Geometry check sheet. Reference: the model listing, model coordinates, mm. A direction names the side the tool comes from. Give positions to 0.01 mm unless a question says otherwise; leave off trailing zeros. Loops run counter-clockwise (first coordinate to the right, second up) from the corner with the lowest first, then second, coordinate; pieces in that order, holes last.
1. Material ranges on L1, parallel to X at y = -34.5, z = 36.65; L2, parallel to X at y = -30.5, z = 7; L3, parallel to Z at x = 5, y = -35, recorded low to high.
2. Cross-section at D-D, the plane y = -4. Record the cut outline in (x, z), plus the area to 3 significant figures.
3. Go/stop test with flat-tipped pins: pin 1 Ø1 at (y, z) = (-33.5, 37) entering from -X; pin 2 Ø2.5 at (x, z) = (36.65, 36.65) entering from +Y. Record where each tip stops, or that it passes through.
4. Cross-section at B-B, the plane z = 21.15. Record the cut outline in (x, y), plus the area to 3 significant figures.
5. Cross-section at C-C, the plane x = 33.5. Record the cut outline in (y, z).
6. Cross-section at A-A, the plane y = -35.5. Record the cut outline in (x, z).
7. Tool access check on faces 4 (the flat face through (0, -19, 21)), 5 (the cylindrical face through (13.04, -39.49, 28.58)). Record the directions out of +Z, -Z, +X, -X, +Y, -Y that give a thin tool (end or side, any length) a straight path to the whole face; none if there is none.
8. Release check for a two-part mould opening along Z. For faces 1 (the flat face through (3, -19, 3)), 2 (the cylindrical face through (5, -33.9, 35.3)), 3 (the flat face through (21, -41, 21)) record: +Z half, -Z half, draft (parallel to the pull), parting line (faces both ways), or undercut.
from build123d import *

# Parameters (mm, degrees)
F0_W     = 42.3
F0_H     = 42.3
F1_DEPTH = 39
F2_R     = 11
F3_DEPTH = 2
F4_SIZE  = 1
F6_D     = 3
F6_DEPTH = 10
F6_TIP   = 0.9012909285
F7_SIZE  = 6


with BuildPart() as f1:
    # F0 (on Front) → F1 (new body)
    with BuildSketch(Plane.XZ):
        with Locations((21.15, 21.15)):
            Rectangle(F0_W, F0_H)
    extrude(amount=F1_DEPTH)

    # F2 (on face) → F3 (join)
    with BuildSketch(Plane.XZ.offset(39)):
        with Locations((21.15, 21.15)):
            Circle(F2_R)
    extrude(amount=F3_DEPTH)

    # F4
    f4_edges = [f1.edges().sort_by_distance(p)[0] for p in [
        (10.15, -41, 21.15),
    ]]
    chamfer(f4_edges, length=F4_SIZE)

    # F6
    with Locations(Plane.XZ.offset(39)):
        with Locations((5.65, 36.65), (36.65, 36.65), (36.65, 5.65), (5.65, 5.65)):
            Hole(F6_D / 2, depth=F6_DEPTH)
            with Locations((0, 0, -(F6_DEPTH + F6_TIP / 2))):  # 118° drill point
                Cone(0, F6_D / 2, F6_TIP, mode=Mode.SUBTRACT)

    # F7
    f7_edges = [f1.edges().sort_by_distance(p)[0] for p in [
        (0, -19.5, 42.3),
        (0, -19.5, 0),
        (42.3, -19.5, 42.3),
        (42.3, -19.5, 0),
    ]]
    chamfer(f7_edges, length=F7_SIZE)


solid = f1.part
Result:
1. L1: x = 0.35 to 4.15, 7.15 to 35.15, 38.15 to 41.95
1. L2: x = 0 to 5, 6.3 to 36, 37.3 to 42.3
1. L3: z = 1 to 4.3, 7 to 35.3, 38 to 41.3
2. outline: (0, 6) - (6, 0) - (36.3, 0) - (42.3, 6) - (42.3, 36.3) - (36.3, 42.3) - (6, 42.3) - (0, 36.3) - close
2. area: 1,720 mm2
3. pin 1: stops at x = 0.2
3. pin 2: stops at y = 0
4. outline: (0, -39) - (10.15, -39) - (10.15, -40) - (11.15, -41) - (31.15, -41) - (32.15, -40) - (32.15, -39) - (42.3, -39) - (42.3, 0) - (0, 0) - close
4. area: 1,690 mm2
5. outline: (-39, 0) - (0, 0) - (0, 42.3) - (-39, 42.3) - close
6. outline: (0, 6) - (6, 0) - (36.3, 0) - (42.3, 6) - (42.3, 36.3) - (36.3, 42.3) - (6, 42.3) - (0, 36.3) - close; hole circle Ø3 at (5.65, 5.65); hole circle Ø3 at (5.65, 36.65); hole circle Ø3 at (36.65, 5.65); hole circle Ø3 at (36.65, 36.65)
7. face 4: +Z, -Z, -X, +Y, -Y
7. face 5: -Y
8. face 1: -Z half
8. face 2: undercut
8. face 3: draft
